```python
from build123d import *

# Parameters (mm, degrees)
SKETCH1_R           = 5
BOSS_EXTRUDE1_DEPTH = 100
SKETCH3_W           = 30
SKETCH3_H           = 30
BOSS_EXTRUDE3_DEPTH = 3
SKETCH4_R           = 1
CUT_EXTRUDE1_DEPTH  = 3


with BuildPart() as part:
    # Sketch1 → Boss-Extrude1 (new body)
    with BuildSketch(Plane(origin=(0, 0, 0), x_dir=(1, 0, 0), z_dir=(0, 1, 0))):
        Circle(SKETCH1_R)
    extrude(amount=BOSS_EXTRUDE1_DEPTH)

    # Sketch3 → Boss-Extrude3 (add)
    with BuildSketch(Plane(origin=(0, 100, 0), x_dir=(1, 0, 0), z_dir=(0, 1, 0))):
        Rectangle(SKETCH3_W, SKETCH3_H)
    extrude(amount=BOSS_EXTRUDE3_DEPTH)

    # Sketch4 → Cut-Extrude1 (cut)
    with BuildSketch(Plane(origin=(0, 103, 0), x_dir=(1, 0, 0), z_dir=(0, 1, 0))):
        with Locations((-13, 13)):
            Circle(SKETCH4_R)
        with Locations((13, 13)):
            Circle(SKETCH4_R)
        with Locations((13, -13)):
            Circle(SKETCH4_R)
        with Locations((-13, -13)):
            Circle(SKETCH4_R)
    extrude(amount=-CUT_EXTRUDE1_DEPTH, mode=Mode.SUBTRACT)

    # Sketch5 → Revolve1 (revolve)
    with BuildSketch(Plane(origin=(0, 0, 0), x_dir=(0, 0, -1), z_dir=(1, 0, 0))):
        Polygon((0, 0), (0, -25), (5, 0), align=None)
    revolve(axis=Axis((0, 0, 0), (0, -1, 0)))


solid = part.part
```
Check sheet for the modelled part. Datum: model origin and axes. Units: mm. A direction names the side the tool comes from. Coordinates: 2 decimals unless noted, no trailing zeros. Write each loop counter-clockwise with the first axis right and the second up, starting at its lowest first coordinate (ties: lowest second). Pieces come first, ordered by that corner, then holes. Notation, with made-up numbers: (55.25, -30.75) - (107.25, -30.75) arc R17 cw to (107.25, -10.75) - close; hole circle Ø3 at (88.25, -19). An arc over 180 degrees is marked (long way). One line per question, with ' | ' between items.
Item 1: Sectioned sample at A-A on y = 88.5. Record the boundary of the cut face in (x, z).
Determined:
outline: circle Ø10 at (0, 0)
Item 2: Thickness scan on line 1 (Z direction, x = 13, y = 101); line 2 (X direction, y = 60.5, z = 0.5). Record the ranges inside material, lowest first. Write a range as [from, to].
Determined:
line 1: z = [-15, -14], [-12, 12], [14, 15] | line 2: x = [-4.97, 4.97]
Item 3: Gauge pin test, flat ends, axial feed: P1, Ø12, axis at x = -11, z = -4, coming from the -Y side; P2, Ø2, axis at x = 5.5, y = 38.5, coming from the +Z side; P3, Ø1.6, axis at x = 13, z = -13, coming from the +Y side; P4, Ø8, axis at y = 86, z = 4.5, coming from the -X side. Record the tip position at first contact, or that the pin passes through.
Determined:
P1: stops at y = 100 | P2: stops at z = 2.18 | P3: passes through | P4: stops at x = -4.97
Item 4: Access from +Z, -Z, +X, -X, +Y, -Y to the whole of each face (thin tool, end or side, straight path). Record for faces 1 (the face through (0, 101, -15)), 2 (the face through (-1.08, 49.3, 4.88)).
Determined:
face 1: -Z, +X, -X, +Y, -Y | face 2: -Y
Item 5: Sectioned sample at C-C on x = 10.25. Record the boundary of the cut face in (y, z).
Determined:
outline: (100, -15) - (103, -15) - (103, 15) - (100, 15) - close
Item 6: Sectioned sample at B-B on z = -6.5. Record the boundary of the cut face in (x, y).
Determined:
outline: (-15, 100) - (15, 100) - (15, 103) - (-15, 103) - close
